Autodesk Inventor part; units mm, degrees
ref_plane "YZ Plane" through (0, 0, 0) normal (1, 0, 0) x (0, 1, 0)
ref_plane "XZ Plane" through (0, 0, 0) normal (0, 1, 0) x (-1, 0, 0)
ref_plane "XY Plane" through (0, 0, 0) normal (0, 0, 1) x (1, 0, 0)
sketch "Sketch1" plane through (0, 0, 0) normal (0, 1, 0) x (-1, 0, 0)
  arc A0 (31.8654, -4.9656) -> (-31.8654, -4.9656) centre (0, 0) ccw
  arc A1 (38.9338, 4.9718) -> (-38.9338, 4.9718) centre (0, 0) ccw
  line L0 (39.25, 0) -> (-39.25, 0)
  line L1 (35.3996, 0) -> (35.3996, 2)
  line L2 (35.3996, 2) -> (35.3996, -2)
  line L3 (36.0047, -4.9656) -> (31.8654, -4.9656)
  line L4 (34.7945, 4.9718) -> (38.9338, 4.9718)
  line L5 (35.3996, 2) -> (34.2752, 2)
  line L6 (34.2752, 2) -> (34.2752, 4.9718)
  line L7 (34.2752, 4.9718) -> (34.7945, 4.9718)
  line L8 (36.0047, -4.9656) -> (36.5241, -4.9656)
  line L9 (36.5241, -4.9656) -> (36.5241, -2)
  line L10 (36.5241, -2) -> (35.3996, -2)
  line L11 (0, 0) -> (0, -17)
  line L12 (-35.3996, 0) -> (-35.3996, 2)
  line L13 (-35.3996, 2) -> (-35.3996, -2)
  line L14 (-36.0047, -4.9656) -> (-31.8654, -4.9656)
  line L15 (-34.7945, 4.9718) -> (-38.9338, 4.9718)
  line L16 (-35.3996, 2) -> (-34.2752, 2)
  line L17 (-34.2752, 2) -> (-34.2752, 4.9718)
  line L18 (-34.2752, 4.9718) -> (-34.7945, 4.9718)
  line L19 (-36.0047, -4.9656) -> (-36.5241, -4.9656)
  line L20 (-36.5241, -4.9656) -> (-36.5241, -2)
  line L21 (-36.5241, -2) -> (-35.3996, -2)
  arc A2 (36.524, -4.9656) -> (36.5241, -4.9651) centre (0, 0) ccw
  arc A3 (36.5232, 4.9718) -> (-36.5232, 4.9718) centre (0, 0) ccw
  arc A4 (-36.5241, -4.9651) -> (-36.524, -4.9656) centre (0, 0) ccw
  dimension "d0" = 64.5
  dimension "d1" = 7
extrude "Extrusion1" add sketch "Sketch1" along normal blind 105 contours A0 L0 L2 L10 L9 L8 L3 | A0 L0 L12 L16 L17 L18 L15 A2 L4 L7 L6 L5 L1 | A0 L14 L19 L20 L21 L13 L0 | A2 L15 A1 L4
chamfer "Chamfer1" distance 0.5 angle 45 6 edges at (36.5241, 52.5, -2) (35.3996, 52.5, 2) (36.5241, 52.5, -4.9656) (-35.3996, 52.5, 2) (-36.5241, 52.5, -2) (-36.5241, 52.5, -4.9656)
extrude "Extrusion2" add sketch "Sketch1" against normal blind 5 contours A2 L15 A1 L4
properties part number "cyl inner"
The listing builds one solid part. Answer for the finished solid, in the listing's coordinates (mm). A direction names the side the tool comes from. Coordinates: 2 decimals unless noted, no trailing zeros. Write each loop counter-clockwise with the first axis right and the second up, starting at its lowest first coordinate (ties: lowest second). Pieces come first, ordered by that corner, then holes. Notation, with made-up numbers: (76.25, 9) - (88.25, 9) arc R32 cw to (88.25, 46) - close; hole circle Ø11 at (7.25, 36.5). An arc over 180 degrees is marked (long way). Return JSON: item names as keys, results as strings. Group by question number.
Q1. Find the intervals of material crossed by line 1 along X through (y, z) = (77, 0); line 2 along Z through (x, y) = (0, 39); line 3 along Y through (x, z) = (28.5, 21.5), in increasing order. Write a range as [from, to].
Q2. The part is cut by section D-D on x = -9. Write down the section's boundary in (y, z), and give its area (3 significant figures).
Q3. The part is cut by section C-C on x = 0. Write down the section's boundary in (y, z), and give its area (3 significant figures).
Q4. Flat-ended cylindrical pins translate along their axes: pin 1 Ø4 at (x, y) = (2, 55.5) entering from -Z; pin 2 Ø4 at (y, z) = (25, 11.5) entering from +X; pin 3 Ø1 at (y, z) = (57.5, -3.5) entering from -X; pin 4 Ø12 at (x, z) = (-24.5, 4) entering from -Y. Find the tip coordinate at first contact, or state that the pin passes through.
Q5. The part is cut by section A-A on z = 0. Write down the section's boundary in (x, y), and give its area (3 significant figures).
Q6. The part is cut by section B-B on y = 79. Write down the section's boundary in (x, z), and give its area (3 significant figures).
Q7. For a pull along X with two mould halves and no side action, classify faces 6 (the flat face through (-37, 51, 4.972)), 7 (the cylindrical face through (-0.793, 50.77, 39.242)), 8 (the cylindrical face through (-0.741, -2.465, 36.853)), 9 (the flat face through (34.275, 52, 3)) as +X half, -X half, draft (parallel to the pull), parting line (faces both ways), or undercut.
Q8. Which of the six approach directions +Z, -Z, +X, -X, +Y, -Y give full straight-line access (tool end or side, diameter ignored) to faces 1 (the flat face through (-34, 52, -4.966)), 2 (the flat face through (-8, 0, 32)), 3 (the flat face through (37, 51, 4.972)), 4 (the flat face through (0.2, -5, 37.4)), 5 (the flat face through (-35.4, 52, 0))?
Evaluation:
{
 "1": {"line 1": "x = [-35.4, -32.25], [32.25, 35.4]", "line 2": "z = [32.25, 39.25]", "line 3": "y = [0, 105]"},
 "2": {"outline": "(-5, 35.74) - (0, 35.74) - (0, 30.97) - (105, 30.97) - (105, 38.2) - (-5, 38.2) - close", "area": "772 mm2"},
 "3": {"outline": "(-5, 36.86) - (0, 36.86) - (0, 32.25) - (105, 32.25) - (105, 39.25) - (-5, 39.25) - close", "area": "747 mm2"},
 "4": {"pin 1": "stops at z = 32", "pin 2": "stops at x = 38.08", "pin 3": "stops at x = -36.52", "pin 4": "passes through"},
 "5": {"outline": "(-35.4, 0) - (-32.25, 0) - (-32.25, 105) - (-35.4, 105) - close; (32.25, 0) - (35.4, 0) - (35.4, 105) - (32.25, 105) - close", "area": "661 mm2"},
 "6": {"outline": "(-38.93, 4.97) - (-34.28, 4.97) - (-34.28, 2) - (-34.9, 2) - (-35.4, 1.5) - (-35.4, -2) - (-36.02, -2) - (-36.52, -2.5) - (-36.52, -4.47) - (-36.02, -4.97) - (-31.87, -4.97) arc R32.25 cw (long way) to (31.87, -4.97) - (36.02, -4.97) - (36.52, -4.47) - (36.52, -2.5) - (36.02, -2) - (35.4, -2) - (35.4, 1.5) - (34.9, 2) - (34.28, 2) - (34.28, 4.97) - (38.93, 4.97) arc R39.25 ccw to start", "area": "781 mm2"},
 "7": {"face 6": "draft", "face 7": "parting line", "face 8": "undercut", "face 9": "+X half"},
 "8": {"face 1": "-Z, +X, -X, +Y, -Y", "face 2": "-Z, -Y", "face 3": "+X, +Y, -Y", "face 4": "+Z, -Z, +X, -X, -Y", "face 5": "-X, +Y, -Y"}
}
